```python
from build123d import *

# Parameters (mm, degrees)
BASE_FLANGE1_DEPTH = 20
SKETCH2_R          = 3.5
CUT_EXTRUDE1_DEPTH = 3
SKETCH3_R          = 3.41681183
CUT_EXTRUDE2_DEPTH = 3
FILLET1_R          = 6


# Sheet-metal steps are written as plain solids
with BuildPart() as part:
    # Sketch1 → Base-Flange1 (new body)
    with BuildSketch(Plane.XY):
        with BuildLine():
            Line((19.18483114, 107.365276831), (69.443546787, 107.365276831))
            ThreePointArc((69.443546787, 107.365276831), (69.725312696, 107.421298009), (69.964219908, 107.580840304))
            Line((69.964219908, 107.580840304), (79.71206519, 117.321886786))
            ThreePointArc((79.71206519, 117.321886786), (80.437479078, 117.806318361), (81.293028401, 117.976420136))
            Line((81.293028401, 117.976420136), (160.367055374, 117.976420136))
            Line((160.367055374, 117.976420136), (160.367055374, 116.476420136))
            Line((160.367055374, 116.476420136), (81.293028401, 116.476420136))
            ThreePointArc((81.293028401, 116.476420136), (81.011262492, 116.420398957), (80.772355281, 116.260856662))
            Line((80.772355281, 116.260856662), (71.024509998, 106.51981018))
            ThreePointArc((71.024509998, 106.51981018), (70.299096111, 106.035378605), (69.443546787, 105.865276831))
            Line((69.443546787, 105.865276831), (19.18483114, 105.865276831))
            Line((19.18483114, 105.865276831), (19.18483114, 107.365276831))
        make_face()
    extrude(amount=BASE_FLANGE1_DEPTH)

    # Sketch2 → Cut-Extrude1 (cut)
    with BuildSketch(Plane(origin=(0, 107.365276831, 0), x_dir=(1, 0, 0), z_dir=(0, 1, 0))):
        with Locations(Location((31.715129554, -10, 0), (0, 0, 270))):
            Circle(SKETCH2_R)
    extrude(amount=-CUT_EXTRUDE1_DEPTH, mode=Mode.SUBTRACT)

    # Sketch3 → Cut-Extrude2 (cut)
    with BuildSketch(Plane(origin=(0, 107.365276831, 0), x_dir=(1, 0, 0), z_dir=(0, 1, 0))):
        with Locations(Location((48.827870371, -10, 0), (0, 0, 270))):
            Circle(SKETCH3_R)
    extrude(amount=-CUT_EXTRUDE2_DEPTH, mode=Mode.SUBTRACT)

    # Fillet1
    fillet1_edges = [part.edges().sort_by_distance(p)[0] for p in [
        (19.18483114, 106.615276831, 0),
        (160.367055374, 117.226420136, 0),
        (19.18483114, 106.615276831, 20),
        (160.367055374, 117.226420136, 20),
    ]]
    fillet(fillet1_edges, radius=FILLET1_R)


solid = part.part
```
Design review of the part built by this model. Coordinates are the model's own, in mm. A direction names the side the tool comes from. Coordinates: 2 decimals unless noted, no trailing zeros. Write each loop counter-clockwise with the first axis right and the second up, starting at its lowest first coordinate (ties: lowest second). Pieces come first, ordered by that corner, then holes.
1) To check wall thickness, follow L1, parallel to X at y = 107.1, z = 10; L2, parallel to X at y = 106.6, z = 10; L3, parallel to Y at x = 117, z = 19. State the ranges of each line that lie inside material, in increasing order.
2) Insertion check: pin 1 (6 mm diameter, centred on x = 119, y = 112, fed in from +Z); pin 2 (11 mm diameter, centred on x = 31.72, z = 10, fed in from +Y); pin 3 (2 mm diameter, centred on y = 109, z = 7.5, fed in from -X); pin 4 (6 mm diameter, centred on y = 111.5, z = 10, fed in from -X). Each pin has a flat end and moves straight along its axis. Give the tip position at first contact, or say it passes through.
3) Add section A-A (z = 10). Write out the cut boundary in (x, y), plus the area to 3 significant figures.
4) Add section B-B (x = 133). Write out the cut boundary in (y, z).
5) Machinability: for faces 1 (the flat face through (44, 107.365, 10)), 2 (the cylindrical face through (20.9, 106.6, 18.2)), 3 (the flat face through (121, 116.476, 10)), which of the approach directions +Z, -Z, +X, -X, +Y, -Y give a long, thin tool a straight path to every point of the face, cutting with its end or side? Answer none if there is none.
6) Add section C-C (y = 111.5). Write out the cut boundary in (x, z).
7) Mouldability with a two-part tool opening along X and no side actions: class faces 4 (the flat face through (74.77, 112.383, 9.86)), 5 (the flat face through (90, 117, 20)), 6 (the cylindrical face through (46.75, 106.63, 7.29)) as +X half, -X half, draft (parallel to the pull), parting line (faces both ways), or undercut.
8) Add section D-D (z = 15.5). Write out the cut boundary in (x, y).
Check result:
1. L1: x = 19.18 to 28.22, 35.22 to 45.41, 52.24 to 71.61
1. L2: x = 19.18 to 28.22, 35.22 to 45.41, 52.24 to 71.1
1. L3: y = 116.48 to 117.98
2. pin 1: passes through
2. pin 2: stops at y = 107.37
2. pin 3: stops at x = 70.38
2. pin 4: stops at x = 70.88
3. outline: (19.18, 105.87) - (28.22, 105.87) - (28.22, 107.37) - (19.18, 107.37) - close; (35.22, 105.87) - (45.41, 105.87) - (45.41, 107.37) - (35.22, 107.37) - close; (52.24, 105.87) - (69.44, 105.87) arc R2.24 ccw to (71.02, 106.52) - (80.77, 116.26) arc R0.74 cw to (81.29, 116.48) - (160.37, 116.48) - (160.37, 117.98) - (81.29, 117.98) arc R2.24 ccw to (79.71, 117.32) - (69.96, 107.58) arc R0.74 cw to (69.44, 107.37) - (52.24, 107.37) - close
3. area: 197 mm2
4. outline: (116.48, 0) - (117.98, 0) - (117.98, 20) - (116.48, 20) - close
5. face 1: +Z, -Z, -X, +Y
5. face 2: +Z, -X, +Y, -Y
5. face 3: +Z, -Z, +X, -Y
6. outline: (73.89, 0) - (76.01, 0) - (76.01, 20) - (73.89, 20) - close
7. face 4: -X half
7. face 5: draft
7. face 6: undercut
8. outline: (19.38, 105.87) - (69.44, 105.87) arc R2.24 ccw to (71.02, 106.52) - (80.77, 116.26) arc R0.74 cw to (81.29, 116.48) - (160.18, 116.48) - (160.18, 117.98) - (81.29, 117.98) arc R2.24 ccw to (79.71, 117.32) - (69.96, 107.58) arc R0.74 cw to (69.44, 107.37) - (19.38, 107.37) - close
